Check sheet for the modelled part. Datum: model origin and axes. Units: mm. A direction names the side the tool comes from. Round coordinates to 2 decimals unless told otherwise and drop trailing zeros. Write each loop counter-clockwise with the first axis right and the second up, starting at its lowest first coordinate (ties: lowest second). Pieces come first, ordered by that corner, then holes.
Item 1: Release check for a two-part mould opening along Y. For faces 1 (the flat face through (81, 39, 100)), 2 (the cylindrical face through (-27.098, -122.028, 49.3)), 3 (the cylindrical face through (72.883, 72.916, 73.794)) record: pulls with the +Y half, pulls with the -Y half, needs draft (parallel to the pull), parting line crosses it, or undercut.
Item 2: Depth check by flat-ended pin: pin 1 (23 mm diameter, centred on y = 90, z = 70, fed in from +X); pin 2 (18.5 mm diameter, centred on x = 0, y = -65, fed in from +Z); pin 3 (8 mm diameter, centred on x = 42, z = 60, fed in from +Y). Enter the tip coordinate at first touch or a pass-through.
Item 3: Section check B-B, the plane y = 90. Record the cut outline in (x, z), plus the area to 3 significant figures.
Item 4: Set-up check for faces 4 (the flat face through (-15, 76, 65)), 5 (the cylindrical face through (-48.53, 28.46, 45.63)), 6 (the cylindrical face through (-0.68, -49.66, 95.06)), 7 (the cylindrical face through (-73.539, 72.916, 73.794)), 8 (the flat face through (43.919, -88.865, 62.467)): record each of +Z, -Z, +X, -X, +Y, -Y from which the full face is reachable in a straight line by a thin tool's end or side.
Item 5: Section check C-C, the plane z = 66. State how many separate pieces and enclosed holes the cut face has, plus the area to 3 significant figures.
Item 6: Material ranges on line 1 along Z through (x, y) = (77, 90); line 2 along X through (y, z) = (-11, 77.5); line 3 along Y through (x, z) = (38, 70), recorded low to high.
from build123d import *

# Parameters (mm, degrees)
BASE_SKETCH_R                            = 125
BASE_EXTRUDE_DEPTH                       = 100
TOP_THRU_HOLE_SKETCH_R                   = 10
SHANK_HOLE_EXTRUDED_CUT_DEPTH            = 204.100960116
OUTER_START                              = -101.827059
SKETCH2_6_R                              = 17.5
SKETCH2_6_R_2                            = 10
OUTER_SLEEVE_EXTRUDED_CUT_DEPTH          = 46.827059
OUTER_START_2                            = 55
TOP_THRU_HOLE_SKETCH_9_R                 = 17.5
OUTER_SLEEVE_EXTRUDED_CUT_2_DEPTH        = 46.827059
SLOTS_START                              = 100
SKETCH1_3_R                              = 32.5
SLOTS_EXTRUDED_CUT_DEPTH                 = 70
FRONT_START                              = 28.831406
SKETCH11_W                               = 30
SKETCH11_H                               = 70
FRONT_SLOT_EXTRUDED_CUT_DEPTH            = 96.168594
CIRCULAR_JAW_PATTERN_COUNT               = 3
COUNTERBORED_HOLE_CIRCULAR_PATTERN_COUNT = 3
CBORE_FOR_M16_HEX_HEAD_BOLT1_AT_2_COUNT  = 2
CBORE_FOR_M16_HEX_HEAD_BOLT1_AT_2_PITCH  = 112.583302492
CBORE_FOR_M16_HEX_HEAD_BOLT1_AT_3_COUNT  = 2
CBORE_FOR_M16_HEX_HEAD_BOLT1_AT_3_PITCH  = 112.583302492


with BuildPart() as part:
    # Base Sketch → Base Extrude (new body)
    with BuildSketch(Plane.XY):
        Circle(BASE_SKETCH_R)
    extrude(amount=BASE_EXTRUDE_DEPTH)

    # Top Thru Hole Sketch → Shank Hole Extruded Cut (cut, symmetric)
    with BuildSketch(Plane(origin=(0, 0, 0), x_dir=(0, 0, -1), z_dir=(1, 0, 0))):
        with Locations((-70, 90)):
            Circle(TOP_THRU_HOLE_SKETCH_R)
    shank_hole_extruded_cut = extrude(amount=SHANK_HOLE_EXTRUDED_CUT_DEPTH, both=True, mode=Mode.SUBTRACT)

    # Sketch2<6> → Outer Sleeve Extruded Cut (cut)
    with BuildSketch(Plane(origin=(0, 0, 0), x_dir=(0, 0, -1), z_dir=(1, 0, 0)).offset(OUTER_START)):
        with Locations((-70, 90)):
            Circle(SKETCH2_6_R)
        with Locations((-70, 90)):
            Circle(SKETCH2_6_R_2, mode=Mode.SUBTRACT)
    outer_sleeve_extruded_cut = extrude(amount=OUTER_SLEEVE_EXTRUDED_CUT_DEPTH, mode=Mode.SUBTRACT)

    # Top Thru Hole Sketch<9> → Outer Sleeve Extruded Cut 2 (cut)
    with BuildSketch(Plane(origin=(0, 0, 0), x_dir=(0, 0, -1), z_dir=(1, 0, 0)).offset(OUTER_START_2)):
        with Locations((-70, 90)):
            Circle(TOP_THRU_HOLE_SKETCH_9_R)
    outer_sleeve_extruded_cut_2 = extrude(amount=OUTER_SLEEVE_EXTRUDED_CUT_2_DEPTH, mode=Mode.SUBTRACT)

    # Sketch1<3> → Slots Extruded Cut (cut)
    with BuildSketch(Plane.XY.offset(SLOTS_START)):
        Circle(SKETCH1_3_R)
    extrude(amount=-SLOTS_EXTRUDED_CUT_DEPTH, mode=Mode.SUBTRACT)

    # Sketch11 → Front Slot Extruded Cut (cut)
    with BuildSketch(Plane(origin=(0, 0, 0), x_dir=(1, 0, 0), z_dir=(0, 1, 0)).offset(FRONT_START)):
        with Locations((0, -65)):
            Rectangle(SKETCH11_W, SKETCH11_H)
    front_slot_extruded_cut = extrude(amount=FRONT_SLOT_EXTRUDED_CUT_DEPTH, mode=Mode.SUBTRACT)

    # Circular Jaw Pattern: Front Slot Extruded Cut ×3 about axis
    circular_jaw_pattern_axis = Axis((0, 0, 0), (0, 0, 1))
    for i in range(1, CIRCULAR_JAW_PATTERN_COUNT):
        add(front_slot_extruded_cut.rotate(circular_jaw_pattern_axis, i * 360 / CIRCULAR_JAW_PATTERN_COUNT), mode=Mode.SUBTRACT)

    # Counterbored Hole Circular Pattern: Shank Hole Extruded Cut, Outer Sleeve Extruded Cut, Outer Sleeve Extruded Cut 2 ×3 about axis
    counterbored_hole_circular_pattern_axis = Axis((0, 0, 0), (0, 0, 1))
    add([shank_hole_extruded_cut.rotate(counterbored_hole_circular_pattern_axis, i * 360 / COUNTERBORED_HOLE_CIRCULAR_PATTERN_COUNT) for i in range(1, COUNTERBORED_HOLE_CIRCULAR_PATTERN_COUNT)], mode=Mode.SUBTRACT)
    add([outer_sleeve_extruded_cut.rotate(counterbored_hole_circular_pattern_axis, i * 360 / COUNTERBORED_HOLE_CIRCULAR_PATTERN_COUNT) for i in range(1, COUNTERBORED_HOLE_CIRCULAR_PATTERN_COUNT)], mode=Mode.SUBTRACT)
    add([outer_sleeve_extruded_cut_2.rotate(counterbored_hole_circular_pattern_axis, i * 360 / COUNTERBORED_HOLE_CIRCULAR_PATTERN_COUNT) for i in range(1, COUNTERBORED_HOLE_CIRCULAR_PATTERN_COUNT)], mode=Mode.SUBTRACT)

    # Sketch15 → CBORE for M16 Hex Head Bolt1 (revolve, cut)
    with BuildSketch(Plane(origin=(56.291651246, 32.5, 100), x_dir=(0, -1, 0), z_dir=(1, 0, 0))):
        Polygon((0, 0), (0, 100), (8.75, 100), (8.75, 10), (15.3565, 10), (15.3565, 0.020977491), (15.3815, 0), align=None)
    cbore_for_m16_hex_head_bolt1 = revolve(axis=Axis((56.291651246, 32.5, 106.35), (0, 0, -1)), mode=Mode.SUBTRACT)

    # CBORE for M16 Hex Head Bolt1 at 2: CBORE for M16 Hex Head Bolt1 ×2
    with Locations(*[Vector(-0.5000000000000011, -0.866025403784438, 0) * (i * CBORE_FOR_M16_HEX_HEAD_BOLT1_AT_2_PITCH) for i in range(1, CBORE_FOR_M16_HEX_HEAD_BOLT1_AT_2_COUNT)]):
        add(cbore_for_m16_hex_head_bolt1, mode=Mode.SUBTRACT)

    # CBORE for M16 Hex Head Bolt1 at 3: CBORE for M16 Hex Head Bolt1 ×2
    with Locations(*[(-i * CBORE_FOR_M16_HEX_HEAD_BOLT1_AT_3_PITCH, 0, 0) for i in range(1, CBORE_FOR_M16_HEX_HEAD_BOLT1_AT_3_COUNT)]):
        add(cbore_for_m16_hex_head_bolt1, mode=Mode.SUBTRACT)


solid = part.part
Values found:
1. face 1: needs draft
1. face 2: parting line crosses it
1. face 3: undercut
2. pin 1: stops at x = 55
2. pin 2: stops at z = 90
2. pin 3: stops at y = 119.08
3. outline: (-86.75, 0) - (86.75, 0) - (86.75, 52.5) - (55, 52.5) - (55, 60) - (15, 60) - (15, 30) - (-15, 30) - (-15, 60) - (-55, 60) - (-55, 52.5) - (-86.75, 52.5) - close; (-86.75, 87.5) - (-55, 87.5) - (-55, 80) - (-15, 80) - (-15, 100) - (-86.75, 100) - close; (15, 80) - (55, 80) - (55, 87.5) - (86.75, 87.5) - (86.75, 100) - (15, 100) - close
3. area: 11,400 mm2
4. face 4: +Z, +Y
4. face 5: +Z, -Z
4. face 6: +Z
4. face 7: -X
4. face 8: none
5. separate pieces: 9
5. enclosed holes: 3
5. area: 26,000 mm2
6. line 1: z = 0 to 52.5, 87.5 to 100
6. line 2: x = -124.52 to -105.21, -89.93 to -49.05, 49.05 to 89.93, 105.21 to 124.52
6. line 3: y = -85.45 to -39.26, -4.62 to 80, 100 to 119.08
